CAD build for the part. Positions are in the model's coordinates, mm. Face numbers are marked on the shaded views. Coordinates: 2 decimals unless noted, no trailing zeros. Loops run counter-clockwise (first coordinate to the right, second up) from the corner with the lowest first, then second, coordinate; pieces in that order, holes last. Notation, with made-up numbers: (37, 41) -> (85, 41) arc R29 ccw to (85, 66) -> close; hole circle Ø7 at (60, 66.5). An arc over 180 degrees is marked (long way). Answer as a JSON object with one key per item and string values. Group by question number.
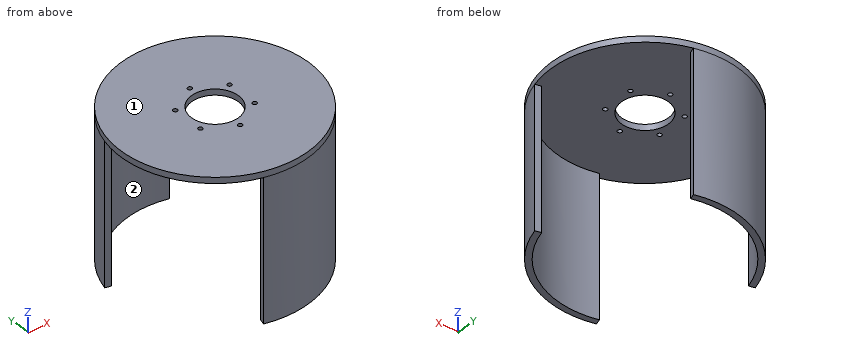
from build123d import *

# Parameters (mm, degrees)
F0_R     = 150
F0_R_2   = 3.4
F0_R_3   = 37.5
F1_DEPTH = 9.525
F3_DEPTH = 225


# Not quite as in the source:
# - a length typed as a fraction of an inch, garbled in the dataset ("3 / 203.2 mm" for 3/8 in), is restored


with BuildPart() as f1:
    # F0 (on Top) → F1 (new body)
    with BuildSketch(Plane.XY):
        Circle(F0_R)
        with Locations((-43.3012701892, -25)):
            Circle(F0_R_2, mode=Mode.SUBTRACT)
        with Locations((0, -50)):
            Circle(F0_R_2, mode=Mode.SUBTRACT)
        with Locations((43.3012701892, -25)):
            Circle(F0_R_2, mode=Mode.SUBTRACT)
        with Locations((-43.3012701892, 25)):
            Circle(F0_R_2, mode=Mode.SUBTRACT)
        Circle(F0_R_3, mode=Mode.SUBTRACT)
        with Locations((43.3012701892, 25)):
            Circle(F0_R_2, mode=Mode.SUBTRACT)
        with Locations((0, 50)):
            Circle(F0_R_2, mode=Mode.SUBTRACT)
    extrude(amount=F1_DEPTH)

    # F2 (on face) → F3 (join)
    with BuildSketch(Plane(origin=(0, 0, 0), x_dir=(1, 0, 0), z_dir=(0, 0, -1))):
        with BuildLine():
            Line((-135.688430448, -36.3576053608), (-144.8888739434, -38.8228567654))
            ThreePointArc((-144.8888739434, -38.8228567654), (-75, -129.9038105677), (38.8228567654, -144.8888739434))
            Line((38.8228567654, -144.8888739434), (36.3576053608, -135.688430448))
            ThreePointArc((36.3576053608, -135.688430448), (-70.2375, -121.6549185966), (-135.688430448, -36.3576053608))
        make_face()
        with BuildLine():
            ThreePointArc((-36.3576053608, 135.688430448), (70.2375, 121.6549185966), (135.688430448, 36.3576053608))
            Line((135.688430448, 36.3576053608), (144.8888739434, 38.8228567654))
            ThreePointArc((144.8888739434, 38.8228567654), (75, 129.9038105677), (-38.8228567654, 144.8888739434))
            Line((-38.8228567654, 144.8888739434), (-36.3576053608, 135.688430448))
        make_face()
    extrude(amount=F3_DEPTH)


solid = f1.part
Item 1: Flat gauge pins, fed straight in: P1, Ø9, axis at x = 43.3, y = -25, coming from the -Z side; P2, Ø12, axis at x = -67, z = -84.5, coming from the +Y side; P3, Ø2, axis at y = 47.5, z = -122, coming from the -X side; P4, Ø11, axis at x = -43.3, y = -25, coming from the +Z side (3 decimals). Where does each tip first touch, or does it go through?
Item 2: Band-saw the part on C-C, the plane x = 97.5. List the corners of the cut face in (y, z) (3 decimals), and give its area (3 significant figures).
Item 3: Band-saw the part on A-A, the plane z = -44. List the corners of the cut face in (x, y) (3 decimals), and give its area (3 significant figures).
Item 4: Band-saw the part on D-D, the plane y = -123. List the corners of the cut face in (x, z) (3 decimals), and give its area (3 significant figures).
Item 5: Pull direction X, two halves, no side cores. Call the marked faces 1 and 2: +X half, -X half, draft (parallel to the pull), parting line (faces both ways), or undercut.
Item 6: Band-saw the part on B-B, the plane y = 0. List the corners of the cut face in (x, z) (3 decimals).
Item 7: Drill centre lines: L1, parallel to Y at x = 0, z = 7; L2, parallel to Z at x = -1, y = -126 (3 decimals); L3, parallel to Y at x = 30.5, z = -43. Where is each one in solid material? Low to high.
Reply:
{
 "1": {"P1": "z = 0", "P2": "y = 137.04", "P3": "x = -142.61", "P4": "z = 9.525"},
 "2": {"outline": "(-113.99, -225) -> (-101.129, -225) -> (-101.129, 0) -> (113.99, 0) -> (113.99, 9.525) -> (-113.99, 9.525) -> close", "area": "5,070 mm²"},
 "3": {"outline": "(-144.889, 38.823) -> (-135.688, 36.358) arc R140.475 cw to (36.358, 135.688) -> (38.823, 144.889) arc R150 ccw to start; (-38.823, -144.889) arc R150 ccw to (144.889, -38.823) -> (135.688, -36.358) arc R140.475 cw to (-36.358, -135.688) -> close", "area": "4,350 mm²"},
 "4": {"outline": "(-85.855, 0) -> (67.854, 0) -> (67.854, -225) -> (85.855, -225) -> (85.855, 9.525) -> (-85.855, 9.525) -> close", "area": "5,690 mm²"},
 "5": {"face 1": "draft", "face 2": "undercut"},
 "6": {"outline": "(-150, 0) -> (-37.5, 0) -> (-37.5, 9.525) -> (-150, 9.525) -> close; (37.5, 0) -> (150, 0) -> (150, 9.525) -> (37.5, 9.525) -> close"},
 "7": {"L1": "-150 to -53.4, -46.6 to -37.5, 37.5 to 46.6, 53.4 to 150", "L2": "0 to 9.525", "L3": "-146.87 to -137.12, 137.12 to 146.87"}
}
